from build123d import *

# Parameters (mm, degrees)
SKETCH1_W                                 = 50
SKETCH1_H                                 = 50
BOSS_EXTRUDE1_DEPTH                       = 2.5
F_4_40_TAPPED_HOLE1_D                     = 2.2606
F_4_40_TAPPED_HOLE1_DEPTH                 = 5
CSK_FOR_4_FLAT_HEAD_MACHINE_SCREW_2_COUNT = 2
CSK_FOR_4_FLAT_HEAD_MACHINE_SCREW_2_PITCH = 30
CUT_EXTRUDE1_REACH                        = 7
SKETCH6_W                                 = 25
SKETCH6_H                                 = 20
FILLET1_R                                 = 5


with BuildPart() as part:
    # Sketch1 → Boss-Extrude1 (new body, symmetric)
    with BuildSketch(Plane(origin=(0, 0, 0), x_dir=(1, 0, 0), z_dir=(0, 1, 0))):
        Rectangle(SKETCH1_W, SKETCH1_H)
    extrude(amount=BOSS_EXTRUDE1_DEPTH, both=True)

    # #4-40 Tapped Hole1
    with Locations(Plane(origin=(0, 2.5, 0), x_dir=(1, 0, 0), z_dir=(0, 1, 0))):
        with Locations((17, 15), (17, -15)):
            Hole(F_4_40_TAPPED_HOLE1_D / 2, depth=F_4_40_TAPPED_HOLE1_DEPTH)

    # Sketch5 → CSK for #4 Flat Head Machine Screw (100)1 (revolve, cut)
    with BuildSketch(Plane(origin=(-17, -2.5, -15), x_dir=(0, 0, -1), z_dir=(1, 0, 0))):
        Polygon((0, 0), (0, 5), (1.63195, 5), (1.63195, 3.028350774), (2.857490729, 2), (2.857490729, 0), align=None)
    csk_for_4_flat_head_machine_screw_100 = revolve(axis=Axis((-17, -8.85, -15), (0, 1, 0)), mode=Mode.SUBTRACT)

    # CSK for _4 Flat Head Machine Screw _ 2: CSK for #4 Flat Head Machine Screw (100)1 ×2
    with Locations(*[(0, 0, i * CSK_FOR_4_FLAT_HEAD_MACHINE_SCREW_2_PITCH) for i in range(1, CSK_FOR_4_FLAT_HEAD_MACHINE_SCREW_2_COUNT)]):
        add(csk_for_4_flat_head_machine_screw_100, mode=Mode.SUBTRACT)

    # Sketch6 → Cut-Extrude1 (cut, up to next)
    with BuildSketch(Plane(origin=(0, 2.5, 0), x_dir=(1, 0, 0), z_dir=(0, 1, 0)), mode=Mode.PRIVATE) as cut_extrude1_sk1:
        Rectangle(SKETCH6_W, SKETCH6_H)
    cut_extrude1_tool1 = extrude(cut_extrude1_sk1.sketch, amount=-CUT_EXTRUDE1_REACH, mode=Mode.PRIVATE) & part.part
    add(cut_extrude1_tool1.solids().sort_by_distance((0, 2.5, 0))[0], mode=Mode.SUBTRACT)

    # Fillet1
    fillet1_edges = [part.edges().sort_by_distance(p)[0] for p in [
        (12.5, 0, -10),
        (12.5, 0, 10),
        (-12.5, 0, 10),
        (-12.5, 0, -10),
        (-25, 0, -25),
        (25, 0, -25),
        (25, 0, 25),
        (-25, 0, 25),
    ]]
    fillet(fillet1_edges, radius=FILLET1_R)


solid = part.part
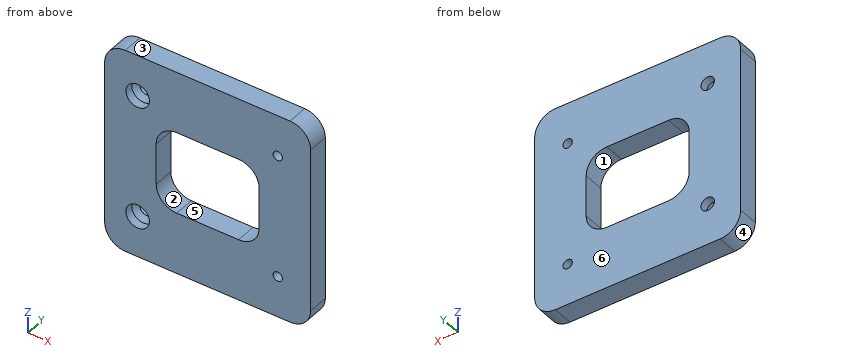
Source: CAD feature listing. Evaluate the final solid. Frame: model axes, mm. Face numbers are marked on the shaded views. A direction names the side the tool comes from. Coordinates: 2 decimals unless noted, no trailing zeros. Order: outer loops, then holes, each group sorted by start corner. A loop starts at its lowest first (then second) coordinate and runs counter-clockwise, first axis right, second up. Notation, with made-up numbers: M 9.5,15 L 66.5,15 A8 ccw 66.5,22 Z; hole C 79,-19.75 d8. An arc over 180 degrees is marked long. Write each question's results on one line, items separated by ' | '. Start each with the question number.
Item 1: Cut plane C-C (y = 1.7). Return loops of the section in (x, z), and give its area (3 significant figures).
Item 2: Set-up query: the marked faces 5 and 6. Return all of +Z, -Z, +X, -X, +Y, -Y with unobstructed straight access to the full face (end or side cutting, diameter ignored); none if empty.
Item 3: Draft query along Z for the marked faces 1, 2, 3 and 4. Return one class per face: pulls with the +Z half, pulls with the -Z half, needs draft (parallel to the pull), parting line crosses it, or undercut.
Item 4: Line query: probe 1 along Z at (x, y) = (-17, 1.1); probe 2 along X at (y, z) = (2, 15); probe 3 along X at (y, z) = (-1.2, 15). Output: solid intervals per line, ascending.
Item 5: Cut plane A-A (z = -15). Return loops of the section in (x, y).
Item 6: Cut plane D-D (x = -1). Return loops of the section in (y, z), and give its area (3 significant figures).
Item 7: Cut plane B-B (x = -17). Return loops of the section in (y, z), and give its area (3 significant figures).
Checked values:
1) outline: M -25,-20 A5 ccw -20,-25 L 20,-25 A5 ccw 25,-20 L 25,20 A5 ccw 20,25 L -20,25 A5 ccw -25,20 Z; hole C -17,-15 d3.26; hole C -17,15 d3.26; hole M -12.5,-5 A5 ccw -7.5,-10 L 7.5,-10 A5 ccw 12.5,-5 L 12.5,5 A5 ccw 7.5,10 L -7.5,10 A5 ccw -12.5,5 Z; hole C 17,-15 d2.26; hole C 17,15 d2.26 | area: 1,980 mm2
2) face 5: +Y, -Y | face 6: +Z, -Z, +X, -X, +Y
3) face 1: undercut | face 2: undercut | face 3: pulls with the +Z half | face 4: pulls with the -Z half
4) probe 1: z = -25 to -16.63, -13.37 to 13.37, 16.63 to 25 | probe 2: x = -25 to -18.63, -15.37 to 15.87, 18.13 to 25 | probe 3: x = -25 to -19.86, -14.14 to 15.87, 18.13 to 25
5) outline: M -25,-2.5 L -19.86,-2.5 L -19.86,-0.5 L -18.63,0.53 L -18.63,2.5 L -25,2.5 Z; M -15.37,0.53 L -14.14,-0.5 L -14.14,-2.5 L 15.87,-2.5 L 15.87,2.5 L -15.37,2.5 Z; M 18.13,-2.5 L 25,-2.5 L 25,2.5 L 18.13,2.5 Z
6) outline: M -2.5,-25 L 2.5,-25 L 2.5,-10 L -2.5,-10 Z; M -2.5,10 L 2.5,10 L 2.5,25 L -2.5,25 Z | area: 150 mm2
7) outline: M -2.5,-25 L 2.5,-25 L 2.5,-16.63 L 0.53,-16.63 L -0.5,-17.86 L -2.5,-17.86 Z; M -2.5,-12.14 L -0.5,-12.14 L 0.53,-13.37 L 2.5,-13.37 L 2.5,13.37 L 0.53,13.37 L -0.5,12.14 L -2.5,12.14 Z; M -2.5,17.86 L -0.5,17.86 L 0.53,16.63 L 2.5,16.63 L 2.5,25 L -2.5,25 Z | area: 205 mm2
